Source: CAD feature listing. Evaluate the final solid. Frame: model axes, mm. Face numbers are marked on the shaded views. A direction names the side the tool comes from. Give positions to 0.01 mm unless a question says otherwise; leave off trailing zeros. Loops run counter-clockwise (first coordinate to the right, second up) from the corner with the lowest first, then second, coordinate; pieces in that order, holes last. Notation, with made-up numbers: M 43.5,59 L 78.5,59 A23 cw 78.5,88 Z; hole C 62.5,24 d8. An arc over 180 degrees is marked long. Answer in a Markdown table with one row per item.
```python
from build123d import *

# Parameters (mm, degrees)
SM_BASE_FLANGE_2_DEPTH = 21.25
HOLE_WIZARD_M3_1_D     = 3.2
SKETCH_24_R            = 3.6
CUT_EXTRUDE_2_DEPTH    = 75.381197221
M4X0_7_1_D             = 3.3
HOLE_WIZARD_M3_2_D     = 3.2
PATTERN_LINEAR_1_COUNT = 3
PATTERN_LINEAR_1_PITCH = 15


# Sheet-metal steps are written as plain solids
with BuildPart() as part:
    # 草圖16 → 基材-凸緣2 (new, symmetric)
    with BuildSketch(Plane.XY):
        with BuildLine():
            Line((40, 0), (0.7366, 0))
            ThreePointArc((0.7366, 0), (0.215745145, 0.215745145), (0, 0.7366))
            Line((0, 0.7366), (0, 55))
            Line((0, 55), (-4, 55))
            Line((-4, 55), (-4, 0.7366))
            ThreePointArc((-4, 0.7366), (-2.61268198, -2.61268198), (0.7366, -4))
            Line((0.7366, -4), (40, -4))
            Line((40, -4), (40, 0))
        make_face()
    extrude(amount=SM_BASE_FLANGE_2_DEPTH, both=True)

    # M3 餘隙孔1 (through all)
    with Locations(Plane(origin=(0, 0, 0), x_dir=(-1, 0, 0), z_dir=(0, 1, 0))):
        with Locations((-27, 18.75), (-11, 3.75), (-11, 18.75), (-27, 3.75)):
            Hole(HOLE_WIZARD_M3_1_D / 2)

    # 草圖24 → 除料-伸長2 (cut, through all)
    with BuildSketch(Plane.XZ.offset(4)):
        with Locations(Location((19, -8.75, 0), (0, 0, 270))):
            Circle(SKETCH_24_R)
    extrude(amount=-CUT_EXTRUDE_2_DEPTH, mode=Mode.SUBTRACT)

    # M4x0.7 螺紋孔1 (through all)
    with Locations(Plane(origin=(0, 0, 0), x_dir=(0, 0, 1), z_dir=(1, 0, 0))):
        with Locations((16.25, -51), (16.25, -31)):
            m4x0_7_1 = Hole(M4X0_7_1_D / 2)

    # M3 餘隙孔2 (through all)
    with Locations(Plane(origin=(0, -4, 0), x_dir=(-1, 0, 0), z_dir=(0, -1, 0))):
        with Locations((-27.5, 8.75), (-10.5, 8.75)):
            Hole(HOLE_WIZARD_M3_2_D / 2)

    # 直線複製排列1: M4x0.7 螺紋孔1 ×3
    with Locations(*[(0, 0, -i * PATTERN_LINEAR_1_PITCH) for i in range(1, PATTERN_LINEAR_1_COUNT)]):
        add(m4x0_7_1, mode=Mode.SUBTRACT)


solid = part.part
```
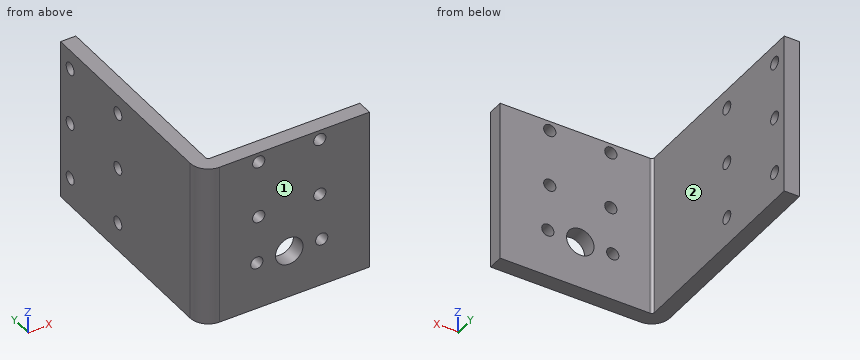
Q1. Ray query, probe 1 along Z at (x, y) = (-2.2, 51); probe 2 along Y at (x, z) = (-1, -13); probe 3 along Z at (x, y) = (27.5, -3.2). Return the intervals inside material, ascending. Write a range as from..to.
Values follow:
| item | result |
|---|---|
| probe 1 | -21.25..-15.4, -12.1..-0.4, 2.9..14.6, 17.9..21.25 |
| probe 2 | -3.67..29.53, 32.47..49.53, 52.47..55 |
| probe 3 | -21.25..-10.35, -7.15..2.23, 5.27..17.23, 20.27..21.25 |
Q2. Section query D-D (z = -13.75). Output: boundary loops of the cut face in (x, y).
Values follow:
| item | result |
|---|---|
| outline | M -4,0.74 A4.74 ccw 0.74,-4 L 40,-4 L 40,0 L 0.74,0 A0.74 cw 0,0.74 L 0,29.35 L -4,29.35 Z; M -4,32.65 L 0,32.65 L 0,49.35 L -4,49.35 Z; M -4,52.65 L 0,52.65 L 0,55 L -4,55 Z |
Q3. Contact query for flat-ended pins moving along their axis: pin 1 Ø1.5 at (y, z) = (32, 15) entering from +X; pin 2 Ø5 at (x, z) = (11, 18.75) entering from +Y. Output: stop coordinate, or through.
Values follow:
| item | result |
|---|---|
| pin 1 | x = 0 |
| pin 2 | y = 0 |
Q4. Section query A-A (z = 18.75). Output: boundary loops of the cut face in (x, y).
Values follow:
| item | result |
|---|---|
| outline | M -4,0.74 A4.74 ccw 0.74,-4 L 9.4,-4 L 9.4,0 L 0.74,0 A0.74 cw 0,0.74 L 0,55 L -4,55 Z; M 12.6,-4 L 25.4,-4 L 25.4,0 L 12.6,0 Z; M 28.6,-4 L 40,-4 L 40,0 L 28.6,0 Z |
Q5. Reachability of the marked faces 1 and 2 from +Z, -Z, +X, -X, +Y, -Y: full face, straight path, thin tool, end or side. Return the list, or none.
Values follow:
| item | result |
|---|---|
| face 1 | +Z, -Z, +X, -X, -Y |
| face 2 | +Z, -Z, +X, +Y |
Q6. Section query C-C (x = 27.5). Output: boundary loops of the cut face in (y, z), plus the area to 3 significant figures.
Values follow:
| item | result |
|---|---|
| outline | M -4,-21.25 L 0,-21.25 L 0,-10.35 L -4,-10.35 Z; M -4,-7.15 L 0,-7.15 L 0,2.23 L -4,2.23 Z; M -4,5.27 L 0,5.27 L 0,17.23 L -4,17.23 Z; M -4,20.27 L 0,20.27 L 0,21.25 L -4,21.25 Z |
| area | 133 mm^2 |
Q7. Section query B-B (y = 51). Output: boundary loops of the cut face in (x, z), plus the area to 3 significant figures.
Values follow:
| item | result |
|---|---|
| outline | M -4,-21.25 L 0,-21.25 L 0,-15.4 L -4,-15.4 Z; M -4,-12.1 L 0,-12.1 L 0,-0.4 L -4,-0.4 Z; M -4,2.9 L 0,2.9 L 0,14.6 L -4,14.6 Z; M -4,17.9 L 0,17.9 L 0,21.25 L -4,21.25 Z |
| area | 130 mm^2 |
